from build123d import *

# Parameters (mm, degrees)
SKETCHREVOLVEGEARBELT01_W       = 10.6
SKETCHREVOLVEGEARBELT01_H       = 6.175697631
TOOTHEXTRUDECUTGEARBELT01_DEPTH = 11.5
CIRPATTERN2_COUNT               = 20
SKETCH6_R                       = 8
BOSS_EXTRUDE1_DEPTH             = 7
BOSS_EXTRUDE2_START             = 1.4
SKETCH7_R                       = 8
BOSS_EXTRUDE2_DEPTH             = 1.4
CUT_EXTRUDE2_DEPTH              = 17.492422502
CUT_EXTRUDE2_DEPTH_BACK         = 17.492422502
SKETCH8_R                       = 4


with BuildPart() as part:
    # SketchRevolveGearBelt01 → GearBelt01 (revolve)
    with BuildSketch(Plane(origin=(0, 0, 0), x_dir=(0, 0, -1), z_dir=(1, 0, 0)), mode=Mode.PRIVATE) as gearbelt01_sk:
        with Locations((5.3, 3.087848816)):
            Rectangle(SKETCHREVOLVEGEARBELT01_W, SKETCHREVOLVEGEARBELT01_H)
    revolve(gearbelt01_sk.sketch.rotate(Axis((0, 0, 0), (0, 0, -1)), 90), axis=Axis((0, 0, 0), (0, 0, -1)))

    # SketchToothGearBelt01 → ToothExtrudeCutGearBelt01 (cut)
    with BuildSketch(Plane.XY):
        with BuildLine():
            Line((-0.791218763, 6.124803189), (0, 8.715697593))
            Line((0, 8.715697593), (0.791218763, 6.124803189))
            ThreePointArc((0.791218763, 6.124803189), (0.657587048, 6.084000517), (0.599999991, 5.956697634))
            ThreePointArc((0.599999991, 5.956697634), (0, 5.356697643), (-0.599999991, 5.956697634))
            ThreePointArc((-0.599999991, 5.956697634), (-0.657587048, 6.084000517), (-0.791218763, 6.124803189))
        make_face()
    toothextrudecutgearbelt01 = extrude(amount=-TOOTHEXTRUDECUTGEARBELT01_DEPTH, mode=Mode.SUBTRACT)

    # CirPattern2: ToothExtrudeCutGearBelt01 ×20 about axis
    cirpattern2_axis = Axis((0, 0, 0), (0, 0, 1))
    for i in range(1, CIRPATTERN2_COUNT):
        add(toothextrudecutgearbelt01.rotate(cirpattern2_axis, i * 360 / CIRPATTERN2_COUNT), mode=Mode.SUBTRACT)

    # Sketch6 → Boss-Extrude1 (add)
    with BuildSketch(Plane.XY):
        Circle(SKETCH6_R)
    extrude(amount=BOSS_EXTRUDE1_DEPTH)

    # Sketch7 → Boss-Extrude2 (add)
    with BuildSketch(Plane(origin=(0, 0, -10.6), x_dir=(-1, 0, 0), z_dir=(0, 0, -1)).offset(BOSS_EXTRUDE2_START)):
        with Locations(Location((0, 0, 0), (0, 0, 180))):
            Circle(SKETCH7_R)
    extrude(amount=-BOSS_EXTRUDE2_DEPTH)

    # Sketch8 → Cut-Extrude2 (cut, two sides: drawn at the far end of the back side and taken through both)
    with BuildSketch(Plane.XY.offset(-CUT_EXTRUDE2_DEPTH_BACK)):
        Circle(SKETCH8_R)
    extrude(amount=CUT_EXTRUDE2_DEPTH + CUT_EXTRUDE2_DEPTH_BACK, mode=Mode.SUBTRACT)


solid = part.part
For this review, take the finished solid that the model builds, in its own axes (mm). A direction names the side the tool comes from. Give positions to 0.01 mm unless a question says otherwise; leave off trailing zeros. Loops run counter-clockwise (first coordinate to the right, second up) from the corner with the lowest first, then second, coordinate; pieces in that order, holes last. Notation, with made-up numbers: M -16.5,68 L -7.5,68 A14 ccw -7.5,76 Z; hole C -6.75,-7.75 d6. An arc over 180 degrees is marked long. Put each result on its own line as item: value. Start each with the question number.
(1) Wall thickness on L1, parallel to X at y = 0, z = -1; L2, parallel to Z at x = -6.75, y = 1.25: over which ranges is each line inside the solid? List them lowest first.
(2) For pin 1 (4 mm diameter, centred on x = -3, z = -5.5, fed in from +Y); pin 2 (8 mm diameter, centred on y = -2.5, z = -3.5, fed in from +X); pin 3 (1.5 mm diameter, centred on y = -3.5, z = -4, fed in from -X), all flat-tipped, find the tip position at first contact; note any pin that passes through.
(3) The part is to be moulded in two halves that separate along Z. For faces 1 (the flat face through (-4, -2, 7)), 2 (the cylindrical face through (-0.867, -3.905, -2.633)), 3 (the cylindrical face through (4.3, -3.2, -5.2)), say which applies: +Z half, -Z half, draft (parallel to the pull), parting line (faces both ways), or undercut.
(4) Add section D-D, the plane y = 6.5. Write out the cut boundary in (x, z).
(5) Add section A-A, the plane x = -1.75. Write out the cut boundary in (y, z), then the cut area to 3 significant figures.
(6) Machinability: for faces 4 (the cylindrical face through (4.34, 3.14, -5.23)), 5 (the cylindrical face through (5.357, -0.013, -5.226)), 6 (the cylindrical face through (-0.013, -5.357, -5.226)), 7 (the cylindrical face through (0.013, 5.357, -5.226)), which of the approach directions +Z, -Z, +X, -X, +Y, -Y give a long, thin tool a straight path to every point of the face, cutting with its end or side? Answer none if there is none.
(7) Add section C-C, the plane z = 5.5. Write out the cut boundary in (x, y), then the cut area to 3 significant figures.
Result:
1. L1: x = -5.36 to -4, 4 to 5.36
1. L2: z = -12 to -10.6, 0 to 7
2. pin 1: stops at y = 6.09
2. pin 2: stops at x = 7.98
2. pin 3: stops at x = -5.53
3. face 1: +Z half
3. face 2: draft
3. face 3: undercut
4. outline: M -4.66,-12 L 4.66,-12 L 4.66,-10.6 L -4.66,-10.6 Z; M -4.66,0 L 4.66,0 L 4.66,7 L -4.66,7 Z
5. outline: M -7.81,-12 L -3.6,-12 L -3.6,7 L -7.81,7 L -7.81,0 L -5.07,0 L -5.07,-10.6 L -7.81,-10.6 Z; M 3.6,-12 L 7.81,-12 L 7.81,-10.6 L 5.07,-10.6 L 5.07,0 L 7.81,0 L 7.81,7 L 3.6,7 Z
5. area: 102 mm^2
6. face 4: none
6. face 5: +X
6. face 6: -Y
6. face 7: +Y
7. outline: C 0,0 d16; hole C 0,0 d8
7. area: 151 mm^2
